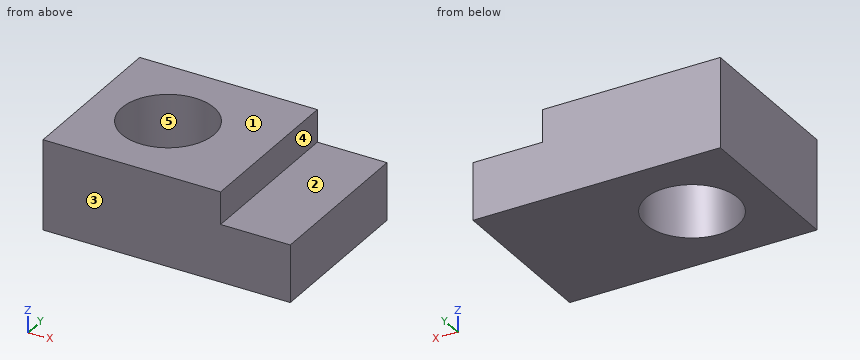
from build123d import *

# Parameters (mm, degrees)
F0_W     = 144.8
F0_H     = 96.4
F1_DEPTH = 33.6
F2_W     = 104
F2_H     = 96.4
F3_DEPTH = 19
F4_R     = 27
F5_DEPTH = 159


with BuildPart() as f1:
    # F0 (on Top) → F1 (new body)
    with BuildSketch(Plane.XY):
        Rectangle(F0_W, F0_H)
    extrude(amount=F1_DEPTH)

    # F2 (on face) → F3 (join)
    with BuildSketch(Plane.XY.offset(33.6)):
        with Locations((-20.4, 0)):
            Rectangle(F2_W, F2_H)
    extrude(amount=F3_DEPTH)

    # F4 (on face) → F5 (cut)
    with BuildSketch(Plane.XY.offset(52.6)):
        with Locations((-27.513253, 0)):
            Circle(F4_R)
    extrude(amount=-F5_DEPTH, mode=Mode.SUBTRACT)


solid = f1.part
Geometry: final body of the model. Coordinates: model frame, mm. Face numbers are marked on the shaded views. A direction names the side the tool comes from. Give positions to 0.01 mm unless a question says otherwise; leave off trailing zeros. Loops run counter-clockwise (first coordinate to the right, second up) from the corner with the lowest first, then second, coordinate; pieces in that order, holes last. Notation, with made-up numbers: (-37, -34.75) -> (4, -34.75) arc R29 ccw to (4, -6.75) -> close; hole circle Ø8 at (9.5, 49.25). An arc over 180 degrees is marked (long way). Put each result on its own line as item: value.
1. Ray query, line 1 along X through (y, z) = (5.5, 45.5); line 2 along Z through (x, y) = (59.5, -11); line 3 along X through (y, z) = (-12, 31). Return the intervals inside material, ascending. Write a range as [from, to].
Taken from the geometry:
line 1: x = [-72.4, -53.95], [-1.08, 31.6]
line 2: z = [0, 33.6]
line 3: x = [-72.4, -51.7], [-3.33, 72.4]
2. Pull-direction query (X, two-part tool) for the marked faces 3, 4 and 5; classes: released by +X, released by -X, zero draft, split by the parting line, or undercut.
Taken from the geometry:
face 3: zero draft
face 4: released by +X
face 5: undercut
3. Pin query (flat end, axial travel): P1, Ø12, axis at y = -31.5, z = 41.5, coming from the +X side. Return the tip coordinate at first contact, or that it passes through.
Taken from the geometry:
P1: stops at x = 31.6
4. Cut plane D-D (y = 18). Return the cut outline in (x, z).
Taken from the geometry:
outline: (-72.4, 0) -> (-47.64, 0) -> (-47.64, 52.6) -> (-72.4, 52.6) -> close; (-7.39, 0) -> (72.4, 0) -> (72.4, 33.6) -> (31.6, 33.6) -> (31.6, 52.6) -> (-7.39, 52.6) -> close
5. Cut plane B-B (z = 30.5). Return the cut outline in (x, y).
Taken from the geometry:
outline: (-72.4, -48.2) -> (72.4, -48.2) -> (72.4, 48.2) -> (-72.4, 48.2) -> close; hole circle Ø54 at (-27.51, 0)
6. Cut plane A-A (y = 0). Return the cut outline in (x, z), plus the area to 3 significant figures.
Taken from the geometry:
outline: (-72.4, 0) -> (-54.51, 0) -> (-54.51, 52.6) -> (-72.4, 52.6) -> close; (-0.51, 0) -> (72.4, 0) -> (72.4, 33.6) -> (31.6, 33.6) -> (31.6, 52.6) -> (-0.51, 52.6) -> close
area: 4,000 mm2
7. Set-up query: the marked faces 1 and 2. Return all of +Z, -Z, +X, -X, +Y, -Y with unobstructed straight access to the full face (end or side cutting, diameter ignored); none if empty.
Taken from the geometry:
face 1: +Z, +X, -X, +Y, -Y
face 2: +Z, +X, +Y, -Y
8. Cut plane C-C (x = -22). Return the cut outline in (y, z).
Taken from the geometry:
outline: (-48.2, 0) -> (-26.43, 0) -> (-26.43, 52.6) -> (-48.2, 52.6) -> close; (26.43, 0) -> (48.2, 0) -> (48.2, 52.6) -> (26.43, 52.6) -> close
